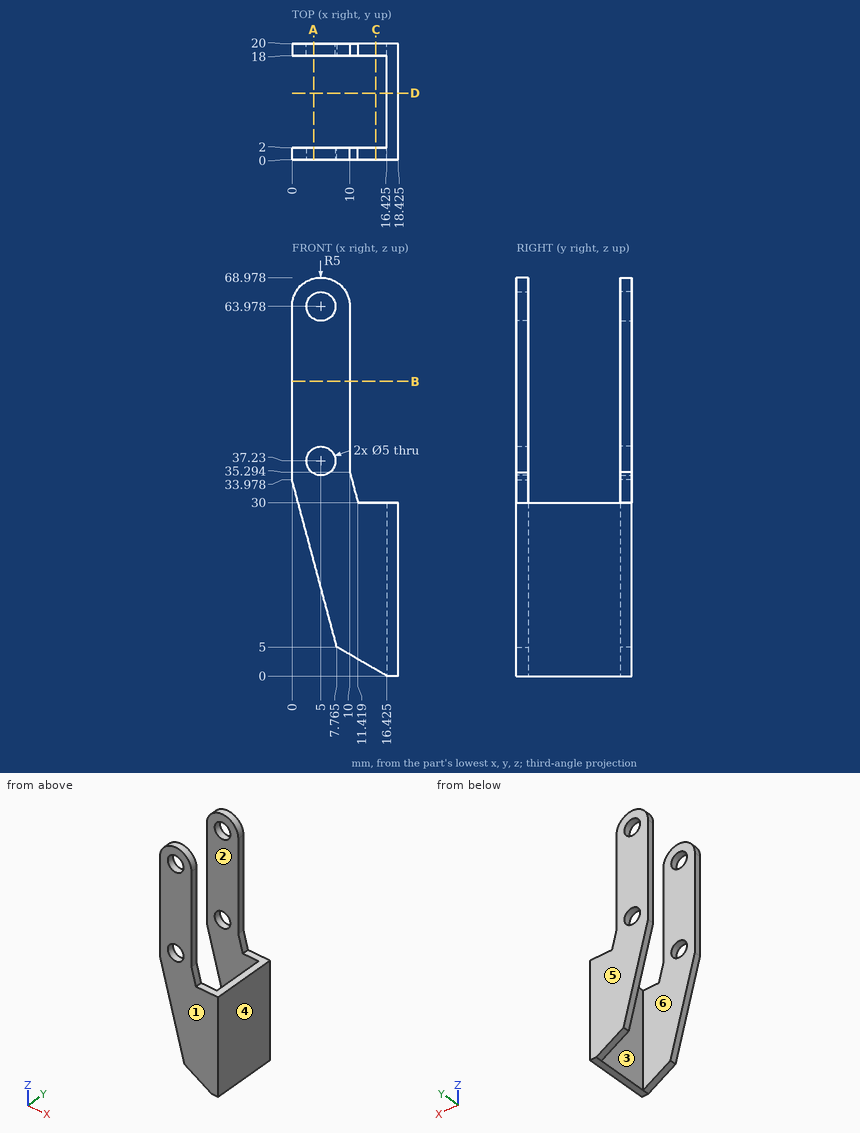
For this review, use the dimensioned drawing (mm, ordinates from the lowest corner) and the shaded views. A direction names the side the tool comes from. Coordinates: 2 decimals unless noted, no trailing zeros. Write each loop counter-clockwise with the first axis right and the second up, starting at its lowest first coordinate (ties: lowest second). Pieces come first, ordered by that corner, then holes. Notation, with made-up numbers: (-10, 43) - (23, 43) arc R26 ccw to (23, 76) - close; hole circle Ø10 at (8.25, 75). An arc over 180 degrees is marked (long way). Answer in a Markdown table with one row per item. Add a question column.
Q1. Consider section B-B on z = 51. Give the boundary of the cut face in (x, y).
Q2. To check wall thickness, follow line 1 along Y through (x, z) = (9, 62.5); line 2 along X through (y, z) = (3.5, 28) (1 decimal). State the ranges of each line that lie inside material, in increasing order. Write a range as from..to.
Q3. Consider section C-C on x = 14.5. Give the boundary of the cut face in (y, z).
Q4. For the marked faces 1 and 2, list the 3-axis set-ups (+Z, -Z, +X, -X, +Y, -Y) from which the entire face can be reached by the end or side of a thin tool; tool diameter is ignored.
Q5. Consider section D-D on y = 11.5. Give the boundary of the cut face in (x, z) (1 decimal).
Q6. Draft analysis for pull direction Y (two halves, no side actions). For the marked faces 3, 4, 5 and 6, state which applies: +Y half, -Y half, draft (parallel to the pull), parting line (faces both ways), or undercut.
Q7. Consider section A-A on x = 3.75. Give the boundary of the cut face in (y, z) (1 decimal), then the cut area to 3 significant figures.
Q8. Clearance check with flat-ended pins moving along their axes: pin 1 (2 mm diameter, centred on y = 19, z = 55, fed in from +X); pin 2 (6.5 mm diameter, centred on x = 5, z = 63.98, fed in from +Y); pin 3 (7.5 mm diameter, centred on x = 16, y = 11.5, fed in from +Z); pin 4 (5 mm diameter, centred on y = 13.5, z = 12, fed in from -X) (1 decimal). State where each tip first meets the part, or that it passes through.
Answers below:
| question | item | result |
|---|---|---|
| 1 | outline | (0, 0) - (10, 0) - (10, 2) - (0, 2) - close; (0, 18) - (10, 18) - (10, 20) - (0, 20) - close |
| 2 | line 1 | 0..2, 18..20 |
| 2 | line 2 | 16.4..18.4 |
| 3 | outline | (0, 1.11) - (2, 1.11) - (2, 30) - (0, 30) - close; (18, 1.11) - (20, 1.11) - (20, 30) - (18, 30) - close |
| 4 | face 1 | +Z, -Z, +X, -X, -Y |
| 4 | face 2 | +Z, -Z, -X |
| 5 | outline | (16.4, 0) - (18.4, 0) - (18.4, 30) - (16.4, 30) - close |
| 6 | face 3 | undercut |
| 6 | face 4 | draft |
| 6 | face 5 | +Y half |
| 6 | face 6 | undercut |
| 7 | outline | (0, 20) - (2, 20) - (2, 35.1) - (0, 35.1) - close; (0, 39.4) - (2, 39.4) - (2, 61.8) - (0, 61.8) - close; (0, 66.1) - (2, 66.1) - (2, 68.8) - (0, 68.8) - close; (18, 20) - (20, 20) - (20, 35.1) - (18, 35.1) - close; (18, 39.4) - (20, 39.4) - (20, 61.8) - (18, 61.8) - close; (18, 66.1) - (20, 66.1) - (20, 68.8) - (18, 68.8) - close |
| 7 | area | 161 mm² |
| 8 | pin 1 | x = 10 |
| 8 | pin 2 | y = 20 |
| 8 | pin 3 | z = 30 |
| 8 | pin 4 | x = 16.4 |
